from build123d import *

# Parameters (mm, degrees)
F0_R     = 50.1
F0_R_2   = 4.5
F1_DEPTH = 3
F2_R     = 7.5
F2_R_2   = 4.5
F3_DEPTH = 10
F4_R     = 1.5


with BuildPart() as f1:
    # F0 (on Front) → F1 (new body)
    with BuildSketch(Plane.XZ):
        Circle(F0_R)
        Circle(F0_R_2, mode=Mode.SUBTRACT)
    extrude(amount=F1_DEPTH)

    # F2 (on face) → F3 (join)
    with BuildSketch(Plane.XZ.offset(3)):
        Circle(F2_R)
        Circle(F2_R_2, mode=Mode.SUBTRACT)
    extrude(amount=F3_DEPTH)

    # F4
    f4_edges = [f1.edges().sort_by_distance(p)[0] for p in [
        (-50.1, 0, 0),
    ]]
    fillet(f4_edges, radius=F4_R)


solid = f1.part
Geometry: final body of the model. Coordinates: model frame, mm. Round coordinates to 2 decimals unless told otherwise and drop trailing zeros. Loops run counter-clockwise (first coordinate to the right, second up) from the corner with the lowest first, then second, coordinate; pieces in that order, holes last.
Q1. Section C-C on y = -4.75. Return loops of the section in (x, z).
Q2. Pin query (flat end, axial travel): P1, Ø2, axis at x = -18.5, z = -8, coming from the -Y side; P2, Ø2, axis at x = 4, y = -10, coming from the +Z side; P3, Ø2, axis at x = -6, y = -1.5, coming from the +Z side. Return the tip coordinate at first contact, or that it passes through.
Q3. Section A-A on z = 0. Return loops of the section in (x, y), plus the area to 3 significant figures.
Q4. Material intervals for L1, parallel to Z at x = 0, y = -5; L2, parallel to Y at x = 10, z = 45; L3, parallel to Z at x = -3.5, y = -1.5, sorted ascending.
Q5. Pull-direction query (Z, two-part tool) for faces 1 (the cylindrical face through (-7.493, -7.93, 0.33)), 2 (the flat face through (-1, 0, -10)), 3 (the cylindrical face through (-0.59, -6.41, 4.46)); classes: released by +Z, released by -Z, zero draft, split by the parting line, or undercut.
Q6. Section B-B on x = 0. Return loops of the section in (y, z).
Evaluation:
1. outline: circle Ø15 at (0, 0); hole circle Ø9 at (0, 0)
2. P1: stops at y = -3
2. P2: stops at z = 6.87
2. P3: stops at z = 49.85
3. outline: (-50.1, -3) - (-7.5, -3) - (-7.5, -13) - (-4.5, -13) - (-4.5, 0) - (-48.6, 0) arc R1.5 ccw to (-50.1, -1.5) - close; (4.5, -13) - (7.5, -13) - (7.5, -3) - (50.1, -3) - (50.1, -1.5) arc R1.5 ccw to (48.6, 0) - (4.5, 0) - close
3. area: 333 mm2
4. L1: z = -7.5 to -4.5, 4.5 to 7.5
4. L2: y = -3 to 0
4. L3: z = -49.98 to -2.83, 2.83 to 49.98
5. face 1: split by the parting line
5. face 2: zero draft
5. face 3: undercut
6. outline: (-13, -7.5) - (-3, -7.5) - (-3, -50.1) - (-1.5, -50.1) arc R1.5 ccw to (0, -48.6) - (0, -4.5) - (-13, -4.5) - close; (-13, 4.5) - (0, 4.5) - (0, 48.6) arc R1.5 ccw to (-1.5, 50.1) - (-3, 50.1) - (-3, 7.5) - (-13, 7.5) - close
